Build history of the part. All positions in model axes, mm. Face numbers are marked on the shaded views. A direction names the side the tool comes from. Round coordinates to 2 decimals unless told otherwise and drop trailing zeros. Write each loop counter-clockwise with the first axis right and the second up, starting at its lowest first coordinate (ties: lowest second). Pieces come first, ordered by that corner, then holes. Notation, with made-up numbers: (-32.5, 74.5) -> (24.5, 74.5) arc R21 ccw to (24.5, 100.5) -> close; hole circle Ø4 at (56.25, 16). An arc over 180 degrees is marked (long way). Answer in a Markdown table with one row per item.
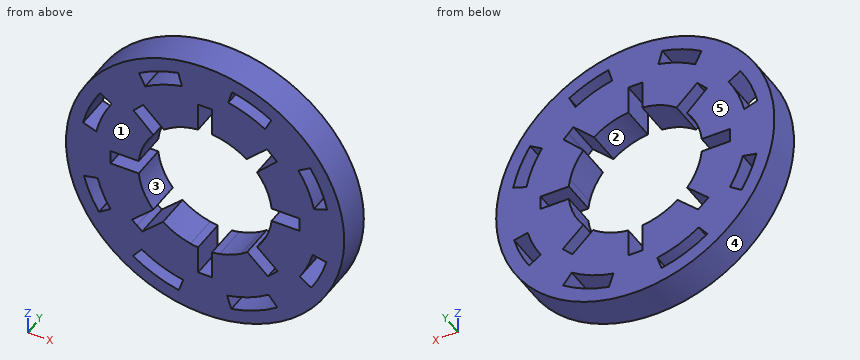
```python
from build123d import *

# Parameters (mm, degrees)
F0_R     = 12.7
F1_DEPTH = 3.175


# Not quite as in the source:
# - ends of sketch curves that miss each other by under 0.0002 mm in the source are joined


with BuildPart() as f1:
    # F0 (on Front) → F1 (new body)
    with BuildSketch(Plane.XZ):
        Circle(F0_R)
        with BuildLine():
            ThreePointArc((11.1424209807, 2.5478137078), (11.3578777025, 1.2819961371), (11.43, 0))
            ThreePointArc((11.43, 0), (11.3372924765, -1.4528245947), (11.0606737878, -2.8820817755))
            ThreePointArc((11.0606737878, -2.8820817755), (10.498054115, -4.5205928591), (9.694266327, -6.0552539485))
            ThreePointArc((9.694266327, -6.0552539485), (8.3067678362, -7.8512742988), (6.5917644701, -9.3377481852))
            ThreePointArc((6.5917644701, -9.3377481852), (4.5881966593, -10.4686843212), (2.3987302505, -11.1754638913))
            ThreePointArc((2.3987302505, -11.1754638913), (0, -11.43), (-2.3987302505, -11.1754638913))
            ThreePointArc((-2.3987302505, -11.1754638913), (-4.5881966593, -10.4686843212), (-6.5917644701, -9.3377481852))
            ThreePointArc((-6.5917644701, -9.3377481852), (-8.3067678362, -7.8512742988), (-9.694266327, -6.0552539485))
            ThreePointArc((-9.694266327, -6.0552539485), (-10.498054115, -4.5205928591), (-11.0606737878, -2.8820817755))
            ThreePointArc((-11.0606737878, -2.8820817755), (-11.4287048944, -0.1720593972), (-11.1424209807, 2.5478137078))
            ThreePointArc((-11.1424209807, 2.5478137078), (-10.5290706386, 4.4478726922), (-9.5944423354, 6.2122118663))
            ThreePointArc((-9.5944423354, 6.2122118663), (-8.0092161617, 8.1545911286), (-6.0386388222, 9.7046247313))
            ThreePointArc((-6.0386388222, 9.7046247313), (-4.3084616277, 10.5868814295), (-2.4538934823, 11.1634809436))
            ThreePointArc((-2.4538934823, 11.1634809436), (0, 11.43), (2.4538934823, 11.1634809436))
            ThreePointArc((2.4538934823, 11.1634809436), (4.3084616277, 10.5868814295), (6.0386388222, 9.7046247313))
            ThreePointArc((6.0386388222, 9.7046247313), (8.0092161617, 8.1545911286), (9.5944423354, 6.2122118663))
            ThreePointArc((9.5944423354, 6.2122118663), (10.5290706386, 4.4478726922), (11.1424209807, 2.5478137078))
        make_face(mode=Mode.SUBTRACT)
        with BuildLine():
            ThreePointArc((10.16, 0), (10.10329164, 1.0719599045), (9.933799599, 2.1319534531))
            ThreePointArc((9.933799599, 2.1319534531), (9.3818599064, 3.8995262145), (8.5182733268, 5.5375644041))
            ThreePointArc((8.5182733268, 5.5375644041), (7.1564472405, 7.2118557178), (5.4717026611, 8.5607283562))
            ThreePointArc((5.4717026611, 8.5607283562), (3.8560932614, 9.3997949318), (2.1166776906, 9.9370657417))
            ThreePointArc((2.1166776906, 9.9370657417), (0, 10.16), (-2.1166776906, 9.9370657417))
            ThreePointArc((-2.1166776906, 9.9370657417), (-3.8560932614, 9.3997949318), (-5.4717026611, 8.5607283562))
            ThreePointArc((-5.4717026611, 8.5607283562), (-7.1564472405, 7.2118557178), (-8.5182733268, 5.5375644041))
            ThreePointArc((-8.5182733268, 5.5375644041), (-9.3818599064, 3.8995262145), (-9.933799599, 2.1319534531))
            ThreePointArc((-9.933799599, 2.1319534531), (-10.1569477884, -0.2490213305), (-9.817387512, -2.6162))
            ThreePointArc((-9.817387512, -2.6162), (-9.3301072422, -4.0217780707), (-8.6427953563, -5.3411317555))
            ThreePointArc((-8.6427953563, -5.3411317555), (-7.3747174058, -6.9885007824), (-5.7978750028, -8.343275463))
            ThreePointArc((-5.7978750028, -8.343275463), (-3.9840291181, -9.3462886744), (-2.0043747759, -9.9603253841))
            ThreePointArc((-2.0043747759, -9.9603253841), (0, -10.16), (2.0043747759, -9.9603253841))
            ThreePointArc((2.0043747759, -9.9603253841), (3.9840291181, -9.3462886744), (5.7978750028, -8.343275463))
            ThreePointArc((5.7978750028, -8.343275463), (7.3747174058, -6.9885007824), (8.6427953563, -5.3411317555))
            ThreePointArc((8.6427953563, -5.3411317555), (9.3301072422, -4.0217780707), (9.817387512, -2.6162))
            ThreePointArc((9.817387512, -2.6162), (10.0739827556, -1.3192692823), (10.16, 0))
        make_face()
        with BuildLine():
            ThreePointArc((4.7360858752, 3.8380602631), (5.4892872515, 2.6512150932), (5.9506155559, 1.323401113))
            Line((5.9506155559, 1.323401113), (8.636, 1.323401113))
            Line((8.636, 1.323401113), (8.636, 0.635))
            Line((8.636, 0.635), (8.636, 0))
            Line((8.636, 0), (8.636, -0.635))
            Line((8.636, -0.635), (8.636, -1.323401113))
            Line((8.636, -1.323401113), (5.9506155559, -1.323401113))
            ThreePointArc((5.9506155559, -1.323401113), (5.6312135784, -2.3346626382), (5.1413854537, -3.2752666482))
            Line((5.1413854537, -3.2752666482), (7.0945855376, -5.080295188))
            Line((7.0945855376, -5.080295188), (6.6273668913, -5.5858669721))
            Line((6.6273668913, -5.5858669721), (5.7343752763, -6.4777944262))
            Line((5.7343752763, -6.4777944262), (5.2671687856, -6.9833774435))
            Line((5.2671687856, -6.9833774435), (3.2744427263, -5.1419102319))
            ThreePointArc((3.2744427263, -5.1419102319), (2.3342114446, -5.631400619), (1.323401113, -5.9506155559))
            Line((1.323401113, -5.9506155559), (1.323401113, -8.636))
            Line((1.323401113, -8.636), (0.635, -8.636))
            Line((0.635, -8.636), (0, -8.636))
            Line((0, -8.636), (-0.635, -8.636))
            Line((-0.635, -8.636), (-1.323401113, -8.636))
            Line((-1.323401113, -8.636), (-1.323401113, -5.9506155559))
            ThreePointArc((-1.323401113, -5.9506155559), (-2.6547777921, -5.4875651135), (-3.8442056919, -4.7310990899))
            Line((-3.8442056919, -4.7310990899), (-5.7343752763, -6.4777944262))
            Line((-5.7343752763, -6.4777944262), (-6.2091766623, -6.0579455764))
            Line((-6.2091766623, -6.0579455764), (-6.6839780483, -5.6380967267))
            Line((-6.6839780483, -5.6380967267), (-4.7360858752, -3.8380602631))
            ThreePointArc((-4.7360858752, -3.8380602631), (-5.6319696302, -2.3328382037), (-6.0628368772, -0.635))
            Line((-6.0628368772, -0.635), (-8.636, -0.635))
            Line((-8.636, -0.635), (-8.636, 0))
            Line((-8.636, 0), (-8.636, 0.635))
            Line((-8.636, 0.635), (-6.0628368772, 0.635))
            ThreePointArc((-6.0628368772, 0.635), (-5.6281633501, 2.3420062564), (-4.7235609165, 3.8534644501))
            Line((-4.7235609165, 3.8534644501), (-6.5416064283, 5.671509962))
            Line((-6.5416064283, 5.671509962), (-6.0925936223, 6.120522768))
            Line((-6.0925936223, 6.120522768), (-5.6552171182, 6.5808778416))
            Line((-5.6552171182, 6.5808778416), (-3.7703908438, 4.7901324496))
            ThreePointArc((-3.7703908438, 4.7901324496), (-2.2927737049, 5.6483984224), (-0.635, 6.0628368772))
            Line((-0.635, 6.0628368772), (-0.635, 8.636))
            Line((-0.635, 8.636), (0, 8.636))
            Line((0, 8.636), (0.635, 8.636))
            Line((0.635, 8.636), (0.635, 6.0628368772))
            ThreePointArc((0.635, 6.0628368772), (2.2927737049, 5.6483984224), (3.7703908438, 4.7901324496))
            Line((3.7703908438, 4.7901324496), (5.6552171182, 6.5808778416))
            Line((5.6552171182, 6.5808778416), (6.0925936223, 6.120522768))
            Line((6.0925936223, 6.120522768), (6.1065741623, 6.1065741623))
            Line((6.1065741623, 6.1065741623), (6.5416223955, 5.6715259292))
            Line((6.5416223955, 5.6715259292), (6.5555869684, 5.6575613563))
            Line((6.5555869684, 5.6575613563), (4.7360858752, 3.8380602631))
        make_face(mode=Mode.SUBTRACT)
        with BuildLine():
            ThreePointArc((11.0606737878, -2.8820817755), (11.3372924765, -1.4528245947), (11.43, 0))
            ThreePointArc((11.43, 0), (11.3578777025, 1.2819961371), (11.1424209807, 2.5478137078))
            Line((11.1424209807, 2.5478137078), (9.933799599, 2.1319534531))
            ThreePointArc((9.933799599, 2.1319534531), (10.10329164, 1.0719599045), (10.16, 0))
            ThreePointArc((10.16, 0), (10.0739827556, -1.3192692823), (9.817387512, -2.6162))
            Line((9.817387512, -2.6162), (11.0606737878, -2.8820817755))
        make_face()
        with BuildLine():
            Line((-9.933799599, 2.1319534531), (-11.1424209807, 2.5478137078))
            ThreePointArc((-11.1424209807, 2.5478137078), (-11.4287048944, -0.1720593972), (-11.0606737878, -2.8820817755))
            Line((-11.0606737878, -2.8820817755), (-9.817387512, -2.6162))
            ThreePointArc((-9.817387512, -2.6162), (-10.1569477884, -0.2490213305), (-9.933799599, 2.1319534531))
        make_face()
        with BuildLine():
            Line((-5.4717026611, 8.5607283562), (-6.0386388222, 9.7046247313))
            ThreePointArc((-6.0386388222, 9.7046247313), (-8.0092161617, 8.1545911286), (-9.5944423354, 6.2122118663))
            Line((-9.5944423354, 6.2122118663), (-8.5182733268, 5.5375644041))
            ThreePointArc((-8.5182733268, 5.5375644041), (-7.1564472405, 7.2118557178), (-5.4717026611, 8.5607283562))
        make_face()
        with BuildLine():
            Line((8.5182733268, 5.5375644041), (9.5944423354, 6.2122118663))
            ThreePointArc((9.5944423354, 6.2122118663), (8.0092161617, 8.1545911286), (6.0386388222, 9.7046247313))
            Line((6.0386388222, 9.7046247313), (5.4717026611, 8.5607283562))
            ThreePointArc((5.4717026611, 8.5607283562), (7.1564472405, 7.2118557178), (8.5182733268, 5.5375644041))
        make_face()
        with BuildLine():
            Line((2.1166776906, 9.9370657417), (2.4538934823, 11.1634809436))
            ThreePointArc((2.4538934823, 11.1634809436), (0, 11.43), (-2.4538934823, 11.1634809436))
            Line((-2.4538934823, 11.1634809436), (-2.1166776906, 9.9370657417))
            ThreePointArc((-2.1166776906, 9.9370657417), (0, 10.16), (2.1166776906, 9.9370657417))
        make_face()
        with BuildLine():
            ThreePointArc((-2.3987302505, -11.1754638913), (0, -11.43), (2.3987302505, -11.1754638913))
            Line((2.3987302505, -11.1754638913), (2.0043747759, -9.9603253841))
            ThreePointArc((2.0043747759, -9.9603253841), (0, -10.16), (-2.0043747759, -9.9603253841))
            Line((-2.0043747759, -9.9603253841), (-2.3987302505, -11.1754638913))
        make_face()
        with BuildLine():
            ThreePointArc((6.5917644701, -9.3377481852), (8.3067678362, -7.8512742988), (9.694266327, -6.0552539485))
            Line((9.694266327, -6.0552539485), (8.6427953563, -5.3411317555))
            ThreePointArc((8.6427953563, -5.3411317555), (7.3747174058, -6.9885007824), (5.7978750028, -8.343275463))
            Line((5.7978750028, -8.343275463), (6.5917644701, -9.3377481852))
        make_face()
        with BuildLine():
            ThreePointArc((-9.694266327, -6.0552539485), (-8.3067678362, -7.8512742988), (-6.5917644701, -9.3377481852))
            Line((-6.5917644701, -9.3377481852), (-5.7978750028, -8.343275463))
            ThreePointArc((-5.7978750028, -8.343275463), (-7.3747174058, -6.9885007824), (-8.6427953563, -5.3411317555))
            Line((-8.6427953563, -5.3411317555), (-9.694266327, -6.0552539485))
        make_face()
        with BuildLine():
            Line((5.7343752763, -6.4777944262), (3.8442056919, -4.7310990899))
            ThreePointArc((3.8442056919, -4.7310990899), (3.565246173, -4.9447179623), (3.2744427263, -5.1419102319))
            Line((3.2744427263, -5.1419102319), (5.2671687856, -6.9833774435))
            Line((5.2671687856, -6.9833774435), (5.7343752763, -6.4777944262))
        make_face()
        with BuildLine():
            Line((1.323401113, -8.636), (1.323401113, -5.9506155559))
            ThreePointArc((1.323401113, -5.9506155559), (0.9808068801, -6.0165799142), (0.635, -6.0628368772))
            Line((0.635, -6.0628368772), (0.635, -8.636))
            Line((0.635, -8.636), (1.323401113, -8.636))
        make_face()
        with BuildLine():
            Line((-0.635, -8.636), (-0.635, -6.0628368772))
            ThreePointArc((-0.635, -6.0628368772), (-0.9808068801, -6.0165799142), (-1.323401113, -5.9506155559))
            Line((-1.323401113, -5.9506155559), (-1.323401113, -8.636))
            Line((-1.323401113, -8.636), (-0.635, -8.636))
        make_face()
        with BuildLine():
            Line((8.636, -0.635), (6.0628368772, -0.635))
            ThreePointArc((6.0628368772, -0.635), (6.0165799142, -0.9808068801), (5.9506155559, -1.323401113))
            Line((5.9506155559, -1.323401113), (8.636, -1.323401113))
            Line((8.636, -1.323401113), (8.636, -0.635))
        make_face()
        with BuildLine():
            ThreePointArc((5.9506155559, 1.323401113), (6.0165799142, 0.9808068801), (6.0628368772, 0.635))
            Line((6.0628368772, 0.635), (8.636, 0.635))
            Line((8.636, 0.635), (8.636, 1.323401113))
            Line((8.636, 1.323401113), (5.9506155559, 1.323401113))
        make_face()
        with BuildLine():
            Line((7.0945855376, -5.080295188), (5.1413854537, -3.2752666482))
            ThreePointArc((5.1413854537, -3.2752666482), (4.9467458118, -3.5624320167), (4.7360858752, -3.8380602631))
            Line((4.7360858752, -3.8380602631), (6.6273668913, -5.5858669721))
            Line((6.6273668913, -5.5858669721), (7.0945855376, -5.080295188))
        make_face()
    extrude(amount=F1_DEPTH)


solid = f1.part
```
Q1. Saw through at D-D on z = 3. Write the cut outline in (x, y) (3 decimals), plus the area to 3 significant figures.
A:
| item | result |
|---|---|
| outline | (-12.341, -3.175) -> (-11.029, -3.175) -> (-11.029, 0) -> (-12.341, 0) -> close; (-9.707, -3.175) -> (-5.307, -3.175) -> (-5.307, 0) -> (-9.707, 0) -> close; (5.307, -3.175) -> (9.707, -3.175) -> (9.707, 0) -> (5.307, 0) -> close; (11.029, -3.175) -> (12.341, -3.175) -> (12.341, 0) -> (11.029, 0) -> close |
| area | 36.3 mm² |
Q2. Drop flat-ended pins along their axis: P1, Ø1.5, axis at x = 2.5, y = -2, coming from the -Z side; P2, Ø1.3, axis at x = 7, y = -1.5, coming from the -Z side; P3, Ø0.8, axis at y = -1, z = 7, coming from the +X side. Give the stop position or say it passes through.
A:
| item | result |
|---|---|
| P1 | z = -12.58 |
| P2 | z = -11 |
| P3 | x = 10.85 |
Q3. Saw through at C-C on x = -3. Write the cut outline in (y, z) (3 decimals), plus the area to 3 significant figures.
A:
| item | result |
|---|---|
| outline | (-3.175, -12.341) -> (0, -12.341) -> (0, -11.029) -> (-3.175, -11.029) -> close; (-3.175, -9.707) -> (0, -9.707) -> (0, -5.307) -> (-3.175, -5.307) -> close; (-3.175, 5.307) -> (0, 5.307) -> (0, 9.707) -> (-3.175, 9.707) -> close; (-3.175, 11.029) -> (0, 11.029) -> (0, 12.341) -> (-3.175, 12.341) -> close |
| area | 36.3 mm² |
Q4. Saw through at A-A on x = 0. Write the cut outline in (y, z) (3 decimals).
A:
| item | result |
|---|---|
| outline | (-3.175, -12.7) -> (0, -12.7) -> (0, -8.636) -> (-3.175, -8.636) -> close; (-3.175, 8.636) -> (0, 8.636) -> (0, 12.7) -> (-3.175, 12.7) -> close |
Q5. Two-plate mould, pull along X, no slides. Class the marked faces 3, 4 and 5: released by +X, released by -X, zero draft, split by the parting line, or undercut.
A:
| item | result |
|---|---|
| face 3 | undercut |
| face 4 | split by the parting line |
| face 5 | zero draft |
Q6. Saw through at B-B on z = 0. Write the cut outline in (x, y) (3 decimals), plus the area to 3 significant figures.
A:
| item | result |
|---|---|
| outline | (-12.7, -3.175) -> (-8.636, -3.175) -> (-8.636, 0) -> (-12.7, 0) -> close; (8.636, -3.175) -> (12.7, -3.175) -> (12.7, 0) -> (8.636, 0) -> close |
| area | 25.8 mm² |
Q7. Wall check: line 1 (Z direction, x = -4.5, y = -0.2); line 2 (Z direction, x = -10.25, y = -1.25); line 3 (X direction, y = -1.4, z = -3.5). Give the ranges that are in metal, low to high. Write a range as [from, to].
A:
| item | result |
|---|---|
| line 1 | [-11.88, -10.51], [-9.11, -5.34], [5.48, 9.11], [10.51, 11.88] |
| line 2 | [-7.5, -5.06], [-2.71, 2.24], [5.06, 7.5] |
| line 3 | [-12.21, -10.88], [-9.54, -4.99], [4.99, 9.54], [10.88, 12.21] |
Q8. Which spindle directions (+Z, -Z, +X, -X, +Y, -Y) get a long thin tool onto all of the face, cutting with end or side? Do the marked faces 1 and 2. Say none if no direction does.
A:
| item | result |
|---|---|
| face 1 | +Z, -Z, +X, -X, -Y |
| face 2 | +Y, -Y |
